Design review of the part built by this model. Coordinates are the model's own, in mm. Face numbers are marked on the shaded views. A direction names the side the tool comes from. Give positions to 0.01 mm unless a question says otherwise; leave off trailing zeros. Write each loop counter-clockwise with the first axis right and the second up, starting at its lowest first coordinate (ties: lowest second). Pieces come first, ordered by that corner, then holes. Notation, with made-up numbers: (-18.5, 37) -> (1.5, 37) arc R24 cw to (1.5, 65) -> close; hole circle Ø6 at (1, 64). An arc over 180 degrees is marked (long way). Use CSV: the item, a comma, the result in double quotes.
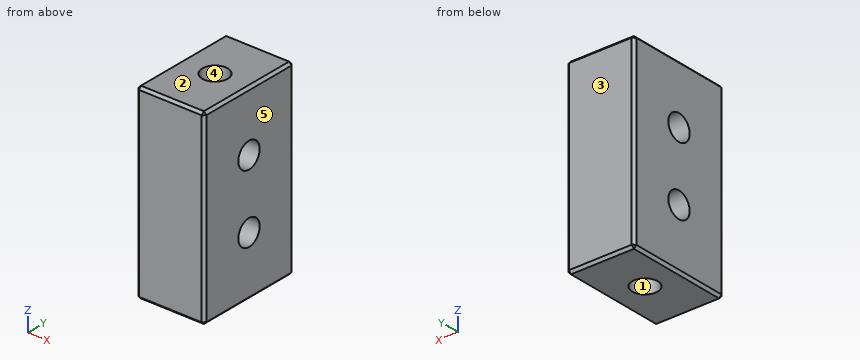
```python
from build123d import *

# Parameters (mm, degrees)
SKETCH_1_W          = 8
SKETCH_1_H          = 12.6
EXTRUDE_1_DEPTH     = 22
CHAMFER_1_SIZE      = 0.3
SKETCH_2_R          = 1.5
CUT_EXTRUDE_1_DEPTH = 25.242318371
SKETCH_3_R          = 1.5
CUT_EXTRUDE_2_DEPTH = 4


with BuildPart() as part:
    # 草图1 → 凸台-拉伸1 (new body)
    with BuildSketch(Plane.XY):
        Rectangle(SKETCH_1_W, SKETCH_1_H)
    extrude(amount=EXTRUDE_1_DEPTH)

    # 倒角1
    chamfer_1_edges = [part.edges().sort_by_distance(p)[0] for p in [
        (-4, 0, 22),
        (0, -6.3, 22),
        (4, 0, 22),
        (0, -6.3, 0),
        (-4, 0, 0),
        (0, 6.3, 0),
        (4, 0, 0),
        (4, -6.3, 11),
        (-4, -6.3, 11),
        (-4, 6.3, 11),
        (4, 6.3, 11),
        (0, 6.3, 22),
    ]]
    chamfer(chamfer_1_edges, length=CHAMFER_1_SIZE)

    # 草图2 → 切除-拉伸1 (cut, through all)
    with BuildSketch(Plane.ZY.offset(4)):
        with Locations(Location((15, 0, 0), (0, 0, 270))):
            Circle(SKETCH_2_R)
        with Locations(Location((7, 0, 0), (0, 0, 90))):
            Circle(SKETCH_2_R)
    extrude(amount=-CUT_EXTRUDE_1_DEPTH, mode=Mode.SUBTRACT)

    # 草图3 → 切除-拉伸2 (cut)
    with BuildSketch(Plane(origin=(0, 0, 0), x_dir=(-1, 0, 0), z_dir=(0, 0, -1))):
        Circle(SKETCH_3_R)
    cut_extrude_2 = extrude(amount=-CUT_EXTRUDE_2_DEPTH, mode=Mode.SUBTRACT)

    # 镜向1: 切除-拉伸2 across plane
    add(cut_extrude_2.mirror(Plane(origin=(0, 0, 11), x_dir=(1, 0, 0), z_dir=(0, 0, -1))), mode=Mode.SUBTRACT)


solid = part.part
```
(1) Take a section at C-C (z = 7). Write out the cut boundary in (x, y), then the cut area to 3 significant figures.
Established:
outline,"(-4, -6) -> (-3.7, -6.3) -> (3.7, -6.3) -> (4, -6) -> (4, -1.5) -> (-4, -1.5) -> close; (-4, 1.5) -> (4, 1.5) -> (4, 6) -> (3.7, 6.3) -> (-3.7, 6.3) -> (-4, 6) -> close"
area,"76.6 mm2"
(2) Tool access review of the marked faces 1 and 2: name each direction out of +Z, -Z, +X, -X, +Y, -Y from which nothing blocks a thin tool from reaching the whole face with its end or side.
Established:
face 1,"-Z"
face 2,"+Z, +X, -X, +Y, -Y"
(3) Take a section at B-B (x = 2.5). Write out the cut boundary in (y, z), then the cut area to 3 significant figures.
Established:
outline,"(-6.3, 0.3) -> (-6, 0) -> (6, 0) -> (6.3, 0.3) -> (6.3, 21.7) -> (6, 22) -> (-6, 22) -> (-6.3, 21.7) -> close; hole circle Ø3 at (0, 7); hole circle Ø3 at (0, 15)"
area,"263 mm2"
(4) Clearance check with flat-ended pins moving along their axes: pin 1 (1.5 mm diameter, centred on x = 0.5, y = 0.5, fed in from +Z); pin 2 (1.8 mm diameter, centred on y = 0, z = 15, fed in from -X); pin 3 (2.5 mm diameter, centred on x = 0, y = 0, fed in from -Z). State where each tip first meets the part, or that it passes through.
Established:
pin 1,"stops at z = 18"
pin 2,"passes through"
pin 3,"stops at z = 4"
(5) Take a section at D-D (x = 0). Write out the cut boundary in (y, z), then the cut area to 3 significant figures.
Established:
outline,"(-6.3, 0.3) -> (-6, 0) -> (-1.5, 0) -> (-1.5, 4) -> (1.5, 4) -> (1.5, 0) -> (6, 0) -> (6.3, 0.3) -> (6.3, 21.7) -> (6, 22) -> (1.5, 22) -> (1.5, 18) -> (-1.5, 18) -> (-1.5, 22) -> (-6, 22) -> (-6.3, 21.7) -> close; hole circle Ø3 at (0, 7); hole circle Ø3 at (0, 15)"
area,"239 mm2"
(6) Mouldability with a two-part tool opening along X and no side actions: class the marked faces 3, 4 and 5 as +X half, -X half, draft (parallel to the pull), parting line (faces both ways), or undercut.
Established:
face 3,"draft"
face 4,"undercut"
face 5,"+X half"
(7) Take a section at A-A (y = 0). Write out the cut boundary in (x, z), then the cut area to 3 significant figures.
Established:
outline,"(-4, 0.3) -> (-3.7, 0) -> (-1.5, 0) -> (-1.5, 4) -> (1.5, 4) -> (1.5, 0) -> (3.7, 0) -> (4, 0.3) -> (4, 5.5) -> (-4, 5.5) -> close; (-4, 8.5) -> (4, 8.5) -> (4, 13.5) -> (-4, 13.5) -> close; (-4, 16.5) -> (4, 16.5) -> (4, 21.7) -> (3.7, 22) -> (1.5, 22) -> (1.5, 18) -> (-1.5, 18) -> (-1.5, 22) -> (-3.7, 22) -> (-4, 21.7) -> close"
area,"104 mm2"
(8) For line 1 along Y through (x, z) = (0, 2.1); line 2 along Z through (x, y) = (-0.75, 0); line 3 along Y through (x, z) = (-2.25, 14.5), list the stretches that pass through material, from the lowest coordinate up. Write a range as [from, to].
Established:
line 1,"y = [-6.3, -1.5], [1.5, 6.3]"
line 2,"z = [4, 5.5], [8.5, 13.5], [16.5, 18]"
line 3,"y = [-6.3, -1.41], [1.41, 6.3]"
